Autodesk Inventor part; units mm, degrees
ref_plane "YZ Plane" through (0, 0, 0) normal (1, 0, 0) x (0, 1, 0)
ref_plane "XZ Plane" through (0, 0, 0) normal (0, 1, 0) x (-1, 0, 0)
ref_plane "XY Plane" through (0, 0, 0) normal (0, 0, 1) x (1, 0, 0)
sketch "Sketch1" plane through (0, 0, 0) normal (0, 1, 0) x (-1, 0, 0)
  circle A0 centre (0, 0) radius 14
  circle A1 centre (0, 0) radius 7.5
  dimension "d0" = 28
  dimension "d1" = 15
extrude "Extrusion1" add sketch "Sketch1" along normal blind 7
sketch "Sketch2" plane through (0, 7, 0) normal (0, 1, 0) x (1, 0, 0)
  line L0 (14, -4) -> (-14, -4)
  line L1 (-14, -4) -> (-14, 4)
  line L2 (-14, 4) -> (14, 4)
  line L3 (14, 4) -> (14, -4)
  line L4 (14, -4) -> (-14, 4) construction
  line L5 (-14, -4) -> (14, 4) construction
  line L6 (-0.5, 5) -> (0.5, 5)
  line L7 (0.5, 5) -> (0.5, -5)
  line L8 (0.5, -5) -> (-0.5, -5)
  line L9 (-0.5, -5) -> (-0.5, 5)
  line L10 (-0.5, 5) -> (0.5, -5) construction
  line L11 (0.5, 5) -> (-0.5, -5) construction
  point P0 (0, 0)
  dimension "d4" = 28
  dimension "d5" = 8
extrude "Extrusion2" cut sketch "Sketch2" against normal blind 8 contours L0 L7 L2 L3 | L0 L9 L2 L7 | L0 L1 L2 L9
sketch "Sketch3" plane through (0, 0, 0) normal (0, -1, 0) x (1, 0, 0)
  circle A0 centre (0, 0) radius 14
  dimension "d17" = 28
extrude "Extrusion3" add sketch "Sketch3" along normal blind 2
sketch "Sketch5" plane through (0, 0, 0) normal (0, 1, 0) x (1, 0, 0)
  point P0 (0, 0)
  point P1 (-0.0372, -0.1116)
hole "Hole2" at (-0.0372, 0, 0.1116) direction (0, -1, 0) diameter 4.5 end through all
extrude "Extrusion4" add sketch "Sketch1" along normal blind 2.5
properties part number "magneticslotV1"
Could you check a few things on this model? Use its own coordinates, in mm. A direction names the side the tool comes from. Round coordinates to 2 decimals unless told otherwise and drop trailing zeros. Loops run counter-clockwise (first coordinate to the right, second up) from the corner with the lowest first, then second, coordinate; pieces in that order, holes last. Notation, with made-up numbers: M 68,46 L 88,46 A4 ccw 88,53 Z; hole C -15,7 d9. An arc over 180 degrees is marked long. Answer as CSV lines item,"result".
1) Imagine slicing it at A-A on y = 4.5. List the corners of the cut face in (x, z) for me.
From the geometry:
outline,"M -13.42,-4 A14 ccw 13.42,-4 L 6.34,-4 A7.5 cw -6.34,-4 Z; M -13.42,4 L -6.34,4 A7.5 cw 6.34,4 L 13.42,4 A14 ccw Z"
2) If I drill on probe 1 along Z at (x, y) = (0, 5); probe 2 along Y at (x, z) = (-12.5, 0.5); probe 3 along X at (y, z) = (2, -3), over which ranges is the centre line in solid material (lowest first)?
From the geometry:
probe 1,"-14 to -7.5, 7.5 to 14"
probe 2,"-2 to 2.5"
probe 3,"-13.67 to -6.87, 6.87 to 13.67"
3) For pin 1 Ø2 at (x, y) = (11.5, 4) entering from -Z; pin 2 Ø1.5 at (y, z) = (2.5, -1) entering from -X; pin 3 Ø1.3 at (x, y) = (10, 5) entering from +Z; pin 4 Ø5 at (x, z) = (1, 6.5) entering from +Y, each with a flat end and sliding along its axis, tell me the tip position at first contact or that it passes through.
From the geometry:
pin 1,"z = -9.26"
pin 2,"x = -14"
pin 3,"z = 10.42"
pin 4,"y = 7"
4) Imagine slicing it at C-C on y = -1. List the corners of the cut face in (x, z) for me.
From the geometry:
outline,"C 0,0 d28; hole C -0.04,0.11 d4.5"
5) Which directions (+Z, -Z, +X, -X, +Y, -Y) give clear straight access to the entire face, cutting with the end or side of a thin tool? Please do faces 1 (the flat face through (0, -2, -3)), 2 (the cylindrical face through (7.493, 1.895, -0.33)), 3 (the flat face through (-10, 5, -4)).
From the geometry:
face 1,"+Z, -Z, +X, -X, -Y"
face 2,"+Y"
face 3,"+X, -X, +Y"
6) We'd pull the mould along X, two halves only. Please class faces 4 (the flat face through (0, 7, -9)), 5 (the flat face through (2, 0, -2)), 6 (the cylindrical face through (-1.934, -1.014, 1.321)): released by +X, released by -X, zero draft, split by the parting line, or undercut.
From the geometry:
face 4,"zero draft"
face 5,"undercut"
face 6,"undercut"
7) Imagine slicing it at B-B on z = -4.75. List the corners of the cut face in (x, y) for me.
From the geometry:
outline,"M -13.17,-2 L 13.17,-2 L 13.17,7 L 5.8,7 L 5.8,0 L -5.8,0 L -5.8,7 L -13.17,7 Z"
